```python
from build123d import *

# Parameters (mm, degrees)
SKETCH_W                           = 164
SKETCH_H                           = 164
PAD_DEPTH                          = 3
SKETCH001_W                        = 164
SKETCH001_H                        = 5
SKETCH001_W_2                      = 5
SKETCH001_H_2                      = 164
PAD001_DEPTH                       = 10
SKETCH005_W                        = 150
SKETCH005_H                        = 2
POCKET_DEPTH                       = 5
SKETCH006_W                        = 150
SKETCH006_H                        = 2
POCKET001_DEPTH                    = 5
SKETCH007_W                        = 2
SKETCH007_H                        = 4
POCKET002_DEPTH                    = 5
LINEARPATTERN_COUNT                = 9
LINEARPATTERN_PITCH                = 17
SKETCH008_W                        = 61.5
SKETCH008_H                        = 3
SKETCH008_W_2                      = 63.5
POCKET003_DEPTH                    = 5
SKETCH009_W                        = 2
SKETCH009_H                        = 4
POCKET004_DEPTH                    = 5
LINEARPATTERN001_COUNT             = 9
LINEARPATTERN001_PITCH             = 17
SKETCH010_W                        = 10
SKETCH010_H                        = 1.8
POCKET005_DEPTH                    = 5
SKETCH010_LINEARPATTERN002_2_W     = 10
SKETCH010_LINEARPATTERN002_2_H     = 1.8
POCKET005_LINEARPATTERN002_2_DEPTH = 5
SKETCH010_LINEARPATTERN002_3_W     = 10
SKETCH010_LINEARPATTERN002_3_H     = 1.8
POCKET005_LINEARPATTERN002_3_DEPTH = 5
SKETCH010_LINEARPATTERN002_4_W     = 10
SKETCH010_LINEARPATTERN002_4_H     = 1.8
POCKET005_LINEARPATTERN002_4_DEPTH = 5
SKETCH010_LINEARPATTERN002_5_W     = 10
SKETCH010_LINEARPATTERN002_5_H     = 1.8
POCKET005_LINEARPATTERN002_5_DEPTH = 5
SKETCH010_LINEARPATTERN002_6_W     = 10
SKETCH010_LINEARPATTERN002_6_H     = 1.8
POCKET005_LINEARPATTERN002_6_DEPTH = 5
SKETCH010_LINEARPATTERN002_7_W     = 10
SKETCH010_LINEARPATTERN002_7_H     = 1.8
POCKET005_LINEARPATTERN002_7_DEPTH = 5
SKETCH010_LINEARPATTERN002_8_W     = 10
SKETCH010_LINEARPATTERN002_8_H     = 1.8
POCKET005_LINEARPATTERN002_8_DEPTH = 5
SKETCH010_LINEARPATTERN002_9_W     = 10
SKETCH010_LINEARPATTERN002_9_H     = 1.8
POCKET005_LINEARPATTERN002_9_DEPTH = 5
LINEARPATTERN003_COUNT             = 2
LINEARPATTERN003_PITCH             = 77
SKETCH011_R                        = 2.5
POCKET006_DEPTH                    = 5
SKETCH012_R                        = 1.5
POCKET007_DEPTH                    = 5
CHAMFER_SIZE                       = 8


with BuildPart() as lb_plate:
    # Sketch → Pad (new body)
    with BuildSketch(Plane.XY):
        Rectangle(SKETCH_W, SKETCH_H)
    extrude(amount=PAD_DEPTH)

    # Sketch001 (on Face6 of Pad) → Pad001 (join)
    with BuildSketch(Plane.XY.offset(3)):
        with Locations((0, -55.5)):
            Rectangle(SKETCH001_W, SKETCH001_H)
        with Locations((-55.5, 0)):
            Rectangle(SKETCH001_W_2, SKETCH001_H_2)
    extrude(amount=PAD001_DEPTH)

    # Sketch005 → Pocket (cut)
    with BuildSketch(Plane(origin=(0, -53, 0), x_dir=(-1, 0, 0), z_dir=(0, 1, 0))):
        with Locations((-7, 12)):
            Rectangle(SKETCH005_W, SKETCH005_H)
    extrude(amount=-POCKET_DEPTH, mode=Mode.SUBTRACT)

    # Sketch006 (on Face15 of Pocket) → Pocket001 (cut)
    with BuildSketch(Plane.YZ.offset(-53)):
        with Locations((7, 12)):
            Rectangle(SKETCH006_W, SKETCH006_H)
    extrude(amount=-POCKET001_DEPTH, mode=Mode.SUBTRACT)

    # Sketch007 (on Face16 of Pocket001) → Pocket002 (cut)
    with BuildSketch(Plane.YZ.offset(-53)):
        with Locations((-37, 9)):
            Rectangle(SKETCH007_W, SKETCH007_H)
    pocket002 = extrude(amount=-POCKET002_DEPTH, mode=Mode.SUBTRACT)

    # LinearPattern: Pocket002 ×9
    with Locations(*[(0, i * LINEARPATTERN_PITCH, 0) for i in range(1, LINEARPATTERN_COUNT)]):
        add(pocket002, mode=Mode.SUBTRACT)

    # Sketch008 (on Face16 of LinearPattern) → Pocket003 (cut)
    with BuildSketch(Plane.YZ.offset(-53)):
        with Locations((-19.25, 4.5)):
            Rectangle(SKETCH008_W, SKETCH008_H)
        with Locations((48.25, 4.5)):
            Rectangle(SKETCH008_W_2, SKETCH008_H)
    extrude(amount=-POCKET003_DEPTH, mode=Mode.SUBTRACT)

    # Sketch009 (on Face19 of Pocket003) → Pocket004 (cut)
    with BuildSketch(Plane(origin=(0, -53, 0), x_dir=(-1, 0, 0), z_dir=(0, 1, 0))):
        with Locations((37, 9)):
            Rectangle(SKETCH009_W, SKETCH009_H)
    pocket004 = extrude(amount=-POCKET004_DEPTH, mode=Mode.SUBTRACT)

    # LinearPattern001: Pocket004 ×9
    with Locations(*[(i * LINEARPATTERN001_PITCH, 0, 0) for i in range(1, LINEARPATTERN001_COUNT)]):
        add(pocket004, mode=Mode.SUBTRACT)

    # Sketch010 (on Face7 of Pocket004) → Pocket005 (cut)
    with BuildSketch(Plane.XY.offset(3)):
        with Locations((1, -37)):
            Rectangle(SKETCH010_W, SKETCH010_H)
    pocket005 = extrude(amount=-POCKET005_DEPTH, mode=Mode.SUBTRACT)

    # Sketch010 LinearPattern002 2 → Pocket005 LinearPattern002 2 (cut)
    with BuildSketch(Plane(origin=(0, 16.9875, 3), x_dir=(1, 0, 0), z_dir=(0, 0, 1))):
        with Locations((1, -37)):
            Rectangle(SKETCH010_LINEARPATTERN002_2_W, SKETCH010_LINEARPATTERN002_2_H)
    pocket005_linearpattern002_2 = extrude(amount=-POCKET005_LINEARPATTERN002_2_DEPTH, mode=Mode.SUBTRACT)

    # Sketch010 LinearPattern002 3 → Pocket005 LinearPattern002 3 (cut)
    with BuildSketch(Plane(origin=(0, 33.975, 3), x_dir=(1, 0, 0), z_dir=(0, 0, 1))):
        with Locations((1, -37)):
            Rectangle(SKETCH010_LINEARPATTERN002_3_W, SKETCH010_LINEARPATTERN002_3_H)
    pocket005_linearpattern002_3 = extrude(amount=-POCKET005_LINEARPATTERN002_3_DEPTH, mode=Mode.SUBTRACT)

    # Sketch010 LinearPattern002 4 → Pocket005 LinearPattern002 4 (cut)
    with BuildSketch(Plane(origin=(0, 50.9625, 3), x_dir=(1, 0, 0), z_dir=(0, 0, 1))):
        with Locations((1, -37)):
            Rectangle(SKETCH010_LINEARPATTERN002_4_W, SKETCH010_LINEARPATTERN002_4_H)
    pocket005_linearpattern002_4 = extrude(amount=-POCKET005_LINEARPATTERN002_4_DEPTH, mode=Mode.SUBTRACT)

    # Sketch010 LinearPattern002 5 → Pocket005 LinearPattern002 5 (cut)
    with BuildSketch(Plane(origin=(0, 67.95, 3), x_dir=(1, 0, 0), z_dir=(0, 0, 1))):
        with Locations((1, -37)):
            Rectangle(SKETCH010_LINEARPATTERN002_5_W, SKETCH010_LINEARPATTERN002_5_H)
    pocket005_linearpattern002_5 = extrude(amount=-POCKET005_LINEARPATTERN002_5_DEPTH, mode=Mode.SUBTRACT)

    # Sketch010 LinearPattern002 6 → Pocket005 LinearPattern002 6 (cut)
    with BuildSketch(Plane(origin=(0, 84.9375, 3), x_dir=(1, 0, 0), z_dir=(0, 0, 1))):
        with Locations((1, -37)):
            Rectangle(SKETCH010_LINEARPATTERN002_6_W, SKETCH010_LINEARPATTERN002_6_H)
    pocket005_linearpattern002_6 = extrude(amount=-POCKET005_LINEARPATTERN002_6_DEPTH, mode=Mode.SUBTRACT)

    # Sketch010 LinearPattern002 7 → Pocket005 LinearPattern002 7 (cut)
    with BuildSketch(Plane(origin=(0, 101.925, 3), x_dir=(1, 0, 0), z_dir=(0, 0, 1))):
        with Locations((1, -37)):
            Rectangle(SKETCH010_LINEARPATTERN002_7_W, SKETCH010_LINEARPATTERN002_7_H)
    pocket005_linearpattern002_7 = extrude(amount=-POCKET005_LINEARPATTERN002_7_DEPTH, mode=Mode.SUBTRACT)

    # Sketch010 LinearPattern002 8 → Pocket005 LinearPattern002 8 (cut)
    with BuildSketch(Plane(origin=(0, 118.9125, 3), x_dir=(1, 0, 0), z_dir=(0, 0, 1))):
        with Locations((1, -37)):
            Rectangle(SKETCH010_LINEARPATTERN002_8_W, SKETCH010_LINEARPATTERN002_8_H)
    pocket005_linearpattern002_8 = extrude(amount=-POCKET005_LINEARPATTERN002_8_DEPTH, mode=Mode.SUBTRACT)

    # Sketch010 LinearPattern002 9 → Pocket005 LinearPattern002 9 (cut)
    with BuildSketch(Plane(origin=(0, 135.9, 3), x_dir=(1, 0, 0), z_dir=(0, 0, 1))):
        with Locations((1, -37)):
            Rectangle(SKETCH010_LINEARPATTERN002_9_W, SKETCH010_LINEARPATTERN002_9_H)
    pocket005_linearpattern002_9 = extrude(amount=-POCKET005_LINEARPATTERN002_9_DEPTH, mode=Mode.SUBTRACT)

    # LinearPattern003: Pocket005, Pocket005 LinearPattern002 2, Pocket005 LinearPattern002 3, Pocket005 LinearPattern002 4, Pocket005 LinearPattern002 5, Pocket005 LinearPattern002 6, Pocket005 LinearPattern002 7, Pocket005 LinearPattern002 8, Pocket005 LinearPattern002 9 ×2
    with Locations(*[(i * LINEARPATTERN003_PITCH, 0, 0) for i in range(1, LINEARPATTERN003_COUNT)]):
        add(pocket005, mode=Mode.SUBTRACT)
        add(pocket005_linearpattern002_2, mode=Mode.SUBTRACT)
        add(pocket005_linearpattern002_3, mode=Mode.SUBTRACT)
        add(pocket005_linearpattern002_4, mode=Mode.SUBTRACT)
        add(pocket005_linearpattern002_5, mode=Mode.SUBTRACT)
        add(pocket005_linearpattern002_6, mode=Mode.SUBTRACT)
        add(pocket005_linearpattern002_7, mode=Mode.SUBTRACT)
        add(pocket005_linearpattern002_8, mode=Mode.SUBTRACT)
        add(pocket005_linearpattern002_9, mode=Mode.SUBTRACT)

    # Sketch011 (on Face155 of MultiTransform) → Pocket006 (cut)
    with BuildSketch(Plane.XZ.offset(58)):
        with Locations((74.5, 7)):
            Circle(SKETCH011_R)
    extrude(amount=-POCKET006_DEPTH, mode=Mode.SUBTRACT)

    # Sketch012 (on Face75 of Pocket006) → Pocket007 (cut)
    with BuildSketch(Plane(origin=(-58, 0, 0), x_dir=(0, -1, 0), z_dir=(-1, 0, 0))):
        with Locations((-73.5, 8.5)):
            Circle(SKETCH012_R)
    extrude(amount=-POCKET007_DEPTH, mode=Mode.SUBTRACT)

    # Chamfer
    chamfer_edges = [lb_plate.edges().sort_by_distance(p)[0] for p in [
        (-82, -55.5, 13),
        (-55.5, -82, 13),
    ]]
    chamfer(chamfer_edges, length=CHAMFER_SIZE)


with BuildPart() as part_mirroring:
    # Part__Mirroring: instance of LB_plate
    add(lb_plate.part.mirror(Plane(origin=(82, 0, 0), x_dir=(0, -1, 0), z_dir=(1, 0, 0))))


solid = part_mirroring.part
```
Input: part model. Units: mm. Frame: model coordinates. A direction names the side the tool comes from. Coordinates: 2 decimals unless noted, no trailing zeros. Write each loop counter-clockwise with the first axis right and the second up, starting at its lowest first coordinate (ties: lowest second). Pieces come first, ordered by that corner, then holes. Notation, with made-up numbers: (28.25, -23.75) -> (48.25, -23.75) arc R19 cw to (48.25, 12.25) -> close; hole circle Ø9 at (-22.5, 66). An arc over 180 degrees is marked (long way). Answer as a JSON object with one key per item and string values.
1. Material intervals for line 1 (Z direction, x = 219.4, y = 73.5); line 2 (Z direction, x = 194, y = 43.5); line 3 (Y direction, x = 142, z = 6), sorted ascending. Write a range as from..to.
Result set:
{"line 1": "z = 0..3, 6..7, 10..11", "line 2": "z = 0..3", "line 3": "y = -58..-53"}
2. Section A-A on y = 35. Return the cut outline in (x, z).
Result set:
{"outline": "(82, 0) -> (246, 0) -> (246, 3) -> (82, 3) -> close; (217, 6) -> (222, 6) -> (222, 11) -> (217, 11) -> close"}
3. Access query for faces 5 (the face through (150, -58, 6)), 6 (the face through (219, -2, 9)), 7 (the face through (234, -70, 3)), 8 (the face through (151, -55, 9)). Directions: +Z, -Z, +X, -X, +Y, -Y. A direction counts if a zero-diameter tool reaches every point of the face in a straight line with its end or side. Return the directions, or none.
Result set:
{"face 5": "+Z, -X, -Y", "face 6": "+Z, +X, -X", "face 7": "+Z, +X, -Y", "face 8": "+Z, +Y, -Y"}
4. First-contact query: P1, Ø4.5, axis at x = 220.5, z = 9.5, coming from the -Y side; P2, Ø0.6, axis at x = 219.5, y = 64.5, coming from the +Z side; P3, Ø6, axis at x = 116.5, z = 9.5, coming from the -Y side. Flat tips, straight axial feed; report the tip coordinate or a pass-through.
Result set:
{"P1": "stops at y = -79.75", "P2": "stops at z = 7", "P3": "stops at y = -58"}
5. Section B-B on x = 153. Return the cut outline in (y, z), then the cut area to 3 significant figures.
Result set:
{"outline": "(-82, 0) -> (82, 0) -> (82, 3) -> (-53, 3) -> (-53, 11) -> (-58, 11) -> (-58, 3) -> (-82, 3) -> close", "area": "532 mm2"}
6. Mould query, pull axis X, two halves, no side actions, for faces 1 (the face through (217, 14, 6)), 2 (the face through (132, -55, 9)), 3 (the face through (246, -1, 1)), 4 (the face through (219, 30, 9)). Classes: released by +X, released by -X, zero draft, split by the parting line, or undercut.
Result set:
{"face 1": "released by -X", "face 2": "undercut", "face 3": "released by +X", "face 4": "zero draft"}
